Source: three-view drawing plus pictorial views. Frame: mm from the lowest corner of the part. Round coordinates to 2 decimals unless told otherwise and drop trailing zeros. Write each loop counter-clockwise with the first axis right and the second up, starting at its lowest first coordinate (ties: lowest second). Pieces come first, ordered by that corner, then holes. Notation, with made-up numbers: M 47.25,-31.75 L 54.25,-31.75 A23 cw 54.25,-14.75 Z; hole C 65.5,-20.5 d9. An arc over 180 degrees is marked long. Answer in a Markdown table with one row per item.
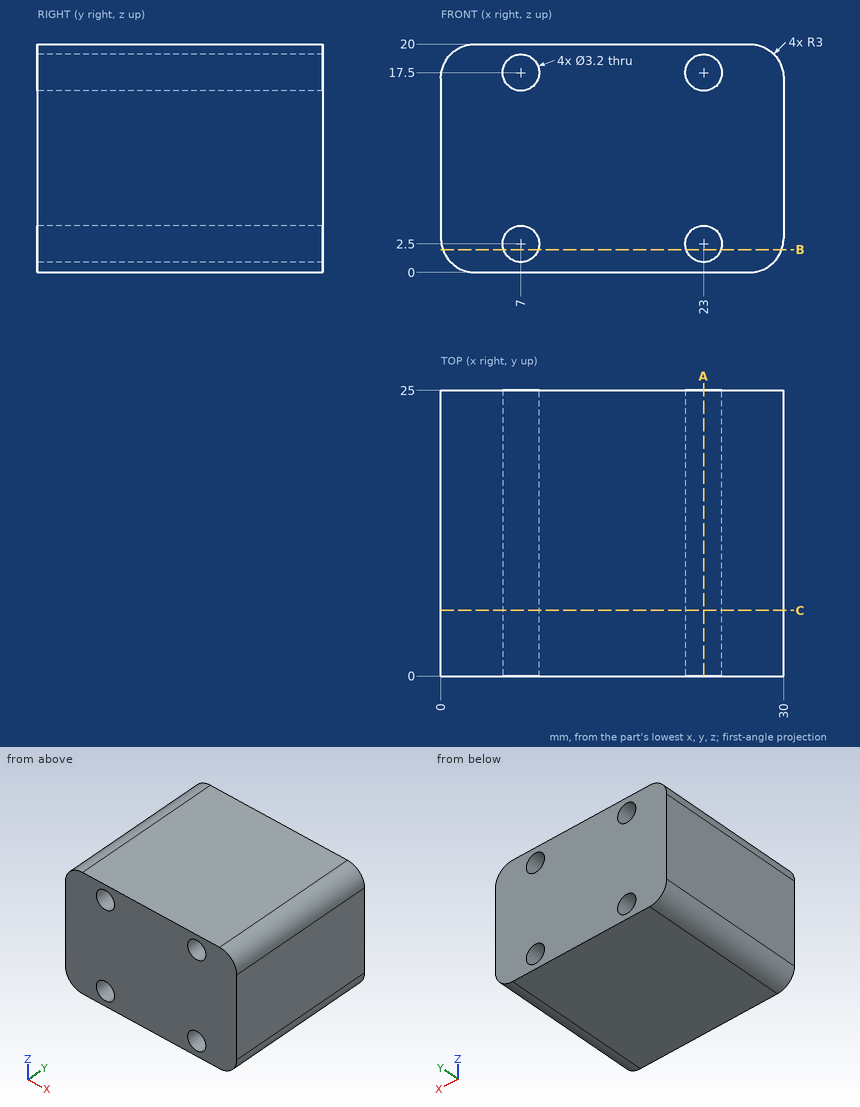
Q1. Section B-B (z = 2). Return loops of the section in (x, y).
Solutions:
| item | result |
|---|---|
| outline | M 0.17,0 L 5.48,0 L 5.48,25 L 0.17,25 Z; M 8.52,0 L 21.48,0 L 21.48,25 L 8.52,25 Z; M 24.52,0 L 29.83,0 L 29.83,25 L 24.52,25 Z |
Q2. Section A-A (x = 23). Return loops of the section in (y, z), and give its area (3 significant figures).
Solutions:
| item | result |
|---|---|
| outline | M 0,0 L 25,0 L 25,0.9 L 0,0.9 Z; M 0,4.1 L 25,4.1 L 25,15.9 L 0,15.9 Z; M 0,19.1 L 25,19.1 L 25,20 L 0,20 Z |
| area | 340 mm2 |
Q3. Material intervals for probe 1 along Z at (x, y) = (23, 19.5); probe 2 along Z at (x, y) = (24, 14); probe 3 along X at (y, z) = (12.5, 2.5), sorted ascending.
Solutions:
| item | result |
|---|---|
| probe 1 | z = 0 to 0.9, 4.1 to 15.9, 19.1 to 20 |
| probe 2 | z = 0 to 1.25, 3.75 to 16.25, 18.75 to 20 |
| probe 3 | x = 0.04 to 5.4, 8.6 to 21.4, 24.6 to 29.96 |
Q4. Contact query for a flat-ended pin moving along its axis: pin 1 Ø3 at (x, z) = (7, 2.5) entering from +Y. Output: stop coordinate, or through.
Solutions:
| item | result |
|---|---|
| pin 1 | passes through |
Q5. Section C-C (y = 5.75). Return loops of the section in (x, z).
Solutions:
| item | result |
|---|---|
| outline | M 0,3 A3 ccw 3,0 L 27,0 A3 ccw 30,3 L 30,17 A3 ccw 27,20 L 3,20 A3 ccw 0,17 Z; hole C 7,2.5 d3.2; hole C 7,17.5 d3.2; hole C 23,2.5 d3.2; hole C 23,17.5 d3.2 |
